Could you check a few things on this model? Use its own coordinates, in mm. A direction names the side the tool comes from. Coordinates: 2 decimals unless noted, no trailing zeros. Write each loop counter-clockwise with the first axis right and the second up, starting at its lowest first coordinate (ties: lowest second). Pieces come first, ordered by that corner, then holes. Notation, with made-up numbers: M 47,-39.5 L 55,-39.5 A17 cw 55,-11.5 Z; hole C 12,-21 d7. An arc over 180 degrees is marked long. Answer as CSV lines item,"result". Start each with the question number.
Item 1: Suppose I cut it at D-D, the plane z = 41. Write out the boundary of the cut face in (x, y).
Item 2: Suppose I cut it at A-A, the plane z = -80.01. Write out the boundary of the cut face in (x, y), and give its area (3 significant figures).
Item 3: If I drill on line 1 along X through (y, z) = (39, -20); line 2 along Z through (x, y) = (1, 32.5); line 3 along Y through (x, z) = (-64, -15), over which ranges is the centre line in solid material (lowest first)? Write a range as [from, to].
Item 4: We'd pull the mould along Z, two halves only. Please class faces 5 (the flat face through (80.01, 24, -59)), 6 (the cylindrical face through (1.013, 7.878, -119.201)), 7 (the flat face through (-1, 21, -123.19)): +Z half, -Z half, draft (parallel to the pull), parting line (faces both ways), or undercut.
Item 5: Suppose I cut it at B-B, the plane x = 46.99. Write out the boundary of the cut face in (y, z), and give its area (3 significant figures).
Item 6: On a 3-axis mill with a long thin cutter (end or side, diameter ignored), from which of +Z, -Z, +X, -X, +Y, -Y can I reach the whole of each face in a straight line? I mean faces 1 (the flat face through (-80.01, 24, -59)), 2 (the flat face through (90.24, 1.88, 115.5)), 3 (the cylindrical face through (-78.722, 23.576, -24.52)), 4 (the flat face through (72.46, 23.88, -3.88)). Say none if no direction works.
Item 7: Suppose I cut it at C-C, the plane y = 18. Write out the boundary of the cut face in (x, z), and give its area (3 significant figures).
Item 8: I'm going to push flat-ended pins straight in: P1, Ø24.5, axis at x = 14.5, y = 23.5, coming from the +Z side; P2, Ø10, axis at y = 29.21, z = -21.59, coming from the +X side; P3, Ø4, axis at y = 36.5, z = -83, coming from the -X side. Where does each tip first touch, or does it pass through?
```python
from build123d import *

# Parameters (mm, degrees)
SKETCH2_W                      = 195.58
SKETCH2_H                      = 246.38
BOSS_EXTRUDE1_DEPTH            = 6.35
FILLET1_R                      = 2.54
SHELL1_START                   = -95.25
SHELL1_OUTLINE_W               = 3.81
SHELL1_OUTLINE_H               = 241.3
SHELL1_DEPTH                   = 190.5
SKETCH3_W                      = 160.02
SKETCH3_H                      = 127
BOSS_EXTRUDE2_DEPTH            = 38.1
FILLET2_R                      = 2.54
SHELL2_START                   = 6.35
SHELL2_OUTLINE_W               = 154.94
SHELL2_OUTLINE_H               = 121.92
SHELL2_DEPTH                   = 35.56
FILLET3_R                      = 5.08
ARDUINO_MOUNT_HOLES_D          = 3.2
CHAMFER1_START                 = 5
CHAMFER1_DEPTH                 = 36.91
TOP_COVER_HOLES_D              = 2.64668
TOP_COVER_HOLES_DEPTH          = 12.7
TOP_COVER_HOLES_TIP            = 0.795142892
CHAMFER2_SIZE                  = 10.16
BOTTOM_COVER_HOLES_D           = 3.81
BOTTOM_COVER_HOLES_DEPTH       = 6.35
BOTTOM_COVER_HOLES_TIP         = 1.144639479
HOLE_FOR_WIRING_D              = 12.7
F_1_2_0_5000_DOWEL_HOLE2_D     = 12.7
F_1_2_0_5000_DOWEL_HOLE2_DEPTH = 2.54
F_1_2_0_5000_DOWEL_HOLE2_TIP   = 3.815464931


with BuildPart() as part:
    # Sketch2 → Boss-Extrude1 (new body)
    with BuildSketch(Plane(origin=(0, 0, 0), x_dir=(1, 0, 0), z_dir=(0, 1, 0))):
        Rectangle(SKETCH2_W, SKETCH2_H)
    extrude(amount=BOSS_EXTRUDE1_DEPTH)

    # Fillet1
    fillet1_edges = [part.edges().sort_by_distance(p)[0] for p in [
        (97.79, 6.35, 0),
        (0, 6.35, -123.19),
        (-97.79, 6.35, 0),
        (-97.79, 3.175, -123.19),
        (97.79, 3.175, -123.19),
        (97.79, 3.175, 123.19),
        (-97.79, 3.175, 123.19),
        (0, 6.35, 123.19),
    ]]
    fillet(fillet1_edges, radius=FILLET1_R)

    # Shell1: read off the stored shape, not the designer's step
    # Shell1 outline → Shell1 (cut)
    with BuildSketch(Plane.YZ.offset(SHELL1_START)):
        with Locations((1.905, 0)):
            Rectangle(SHELL1_OUTLINE_W, SHELL1_OUTLINE_H)
    extrude(amount=SHELL1_DEPTH, mode=Mode.SUBTRACT)

    # Sketch3 → Boss-Extrude2 (add)
    with BuildSketch(Plane(origin=(0, 3.81, 0), x_dir=(-1, 0, 0), z_dir=(0, -1, 0))):
        with Locations((0, 59.69)):
            Rectangle(SKETCH3_W, SKETCH3_H)
    extrude(amount=-BOSS_EXTRUDE2_DEPTH)

    # Fillet2
    fillet2_edges = [part.edges().sort_by_distance(p)[0] for p in [
        (80.01, 22.86, -123.19),
        (-80.01, 22.86, -123.19),
        (80.01, 24.13, 3.81),
        (-80.01, 24.13, 3.81),
    ]]
    fillet(fillet2_edges, radius=FILLET2_R)

    # Shell2: read off the stored shape, not the designer's step
    # Shell2 outline → Shell2 (cut)
    with BuildSketch(Plane(origin=(0, 0, 0), x_dir=(1, 0, 0), z_dir=(0, 1, 0)).offset(SHELL2_START)):
        with Locations((0, 59.69)):
            Rectangle(SHELL2_OUTLINE_W, SHELL2_OUTLINE_H)
    extrude(amount=SHELL2_DEPTH, mode=Mode.SUBTRACT)

    # Fillet3
    fillet3_edges = [part.edges().sort_by_distance(p)[0] for p in [
        (0, 6.35, -120.65),
        (77.47, 6.35, -59.69),
        (-77.47, 6.35, -59.69),
        (0, 6.35, 1.27),
    ]]
    fillet(fillet3_edges, radius=FILLET3_R)

    # Arduino Mount holes (through all)
    with Locations(Plane(origin=(0, 6.35, 0), x_dir=(1, 0, 0), z_dir=(0, 1, 0))):
        with Locations((3.690112, 110.49), (3.690112, 60.4901), (-67.31, 60.4901), (-67.31, 110.49)):
            Hole(ARDUINO_MOUNT_HOLES_D / 2)

    # Chamfer1: read off the stored shape, not the designer's step
    # Chamfer1 outline → Chamfer1 (add)
    with BuildSketch(Plane(origin=(0, 0, 0), x_dir=(1, 0, 0), z_dir=(0, 1, 0)).offset(CHAMFER1_START)):
        Polygon((-77.47, 110.49), (-67.31, 120.65), (-77.47, 120.65), align=None)
        Polygon((77.47, 120.65), (67.31, 120.65), (77.47, 110.49), align=None)
        Polygon((-67.31, -1.27), (-77.47, 8.89), (-77.47, -1.27), align=None)
        Polygon((77.47, -1.27), (77.47, 8.89), (67.31, -1.27), align=None)
    extrude(amount=CHAMFER1_DEPTH)

    # Top cover holes
    with Locations(Plane(origin=(0, 41.91, 0), x_dir=(1, 0, 0), z_dir=(0, 1, 0))):
        with Locations((75.2475, 0.9525), (-75.2475, 0.9525), (-75.2475, 118.4275), (75.2475, 118.4275)):
            Hole(TOP_COVER_HOLES_D / 2, depth=TOP_COVER_HOLES_DEPTH)
            with Locations((0, 0, -(TOP_COVER_HOLES_DEPTH + TOP_COVER_HOLES_TIP / 2))):  # 118° drill point
                Cone(0, TOP_COVER_HOLES_D / 2, TOP_COVER_HOLES_TIP, mode=Mode.SUBTRACT)

    # Chamfer2
    chamfer2_edges = [part.edges().sort_by_distance(p)[0] for p in [
        (-95.25, 1.905, -120.65),
        (-95.25, 1.905, 120.65),
        (95.25, 1.905, 120.65),
        (95.25, 1.905, -120.65),
    ]]
    chamfer(chamfer2_edges, length=CHAMFER2_SIZE)

    # Bottom cover holes
    with Locations(Plane(origin=(0, 0, 0), x_dir=(-1, 0, 0), z_dir=(0, -1, 0))):
        with Locations((-93.0275, 118.4275), (93.0275, 118.4275), (93.0275, -118.4275), (-93.0275, -118.4275)):
            Hole(BOTTOM_COVER_HOLES_D / 2, depth=BOTTOM_COVER_HOLES_DEPTH)
            with Locations((0, 0, -(BOTTOM_COVER_HOLES_DEPTH + BOTTOM_COVER_HOLES_TIP / 2))):  # 118° drill point
                Cone(0, BOTTOM_COVER_HOLES_D / 2, BOTTOM_COVER_HOLES_TIP, mode=Mode.SUBTRACT)

    # Hole for Wiring (through all)
    with Locations(Plane(origin=(0, 6.35, 0), x_dir=(1, 0, 0), z_dir=(0, 1, 0))):
        with Locations((46.99, 80.01)):
            Hole(HOLE_FOR_WIRING_D / 2)

    # 1/2 (0.5000) Dowel Hole2
    with Locations(Plane.ZY.offset(80.01)):
        with Locations((-21.59, 29.21)):
            Hole(F_1_2_0_5000_DOWEL_HOLE2_D / 2, depth=F_1_2_0_5000_DOWEL_HOLE2_DEPTH)
            with Locations((0, 0, -(F_1_2_0_5000_DOWEL_HOLE2_DEPTH + F_1_2_0_5000_DOWEL_HOLE2_TIP / 2))):  # 118° drill point
                Cone(0, F_1_2_0_5000_DOWEL_HOLE2_D / 2, F_1_2_0_5000_DOWEL_HOLE2_TIP, mode=Mode.SUBTRACT)


solid = part.part
```
Ans:
1,outline,"M -97.79,0 L -95.25,0 L -95.25,3.81 L 95.25,3.81 L 95.25,0 L 97.79,0 L 97.79,3.81 A2.54 ccw 95.25,6.35 L -95.25,6.35 A2.54 ccw -97.79,3.81 Z"
2,outline,"M -97.79,0 L -95.25,0 L -95.25,3.81 L 40.64,3.81 L 40.64,6.35 L -72.39,6.35 A5.08 cw -77.47,11.43 L -77.47,41.91 L -80.01,41.91 L -80.01,6.35 L -95.25,6.35 A2.54 ccw -97.79,3.81 Z; M 53.34,3.81 L 95.25,3.81 L 95.25,0 L 97.79,0 L 97.79,3.81 A2.54 ccw 95.25,6.35 L 80.01,6.35 L 80.01,41.91 L 77.47,41.91 L 77.47,11.43 A5.08 cw 72.39,6.35 L 53.34,6.35 Z"
2,area,"673 mm^2"
3,line 1,"x = [-80.01, -77.47], [77.47, 80.01]"
3,line 2,"z = [-123.19, -120.65], [1.27, 3.81]"
3,line 3,"y = [3.81, 6.35]"
4,face 5,"draft"
4,face 6,"undercut"
4,face 7,"-Z half"
5,outline,"M 0,-123.19 L 41.91,-123.19 L 41.91,-120.65 L 11.43,-120.65 A5.08 cw 6.35,-115.57 L 6.35,-86.36 L 3.81,-86.36 L 3.81,-120.65 L 0,-120.65 Z; M 0,120.65 L 3.81,120.65 L 3.81,-73.66 L 6.35,-73.66 L 6.35,-3.81 A5.08 cw 11.43,1.27 L 41.91,1.27 L 41.91,3.81 L 6.35,3.81 L 6.35,120.65 A2.54 ccw 3.81,123.19 L 0,123.19 Z"
5,area,"803 mm^2"
6,face 1,"+Z, -Z, -X, +Y"
6,face 2,"-Y"
6,face 3,"-X"
6,face 4,"+Y"
7,outline,"M -80.01,-120.65 A2.54 ccw -77.47,-123.19 L 77.47,-123.19 A2.54 ccw 80.01,-120.65 L 80.01,1.27 A2.54 ccw 77.47,3.81 L -77.47,3.81 A2.54 ccw -80.01,1.27 Z; hole M -77.47,-110.49 L -67.31,-120.65 L 67.31,-120.65 L 77.47,-110.49 L 77.47,-8.89 L 67.31,1.27 L -67.31,1.27 L -77.47,-8.89 Z"
7,area,"1,630 mm^2"
8,P1,"stops at z = 3.81"
8,P2,"stops at x = 80.01"
8,P3,"stops at x = -80.01"
